from build123d import *

# Parameters (mm, degrees)
SKETCH1_R           = 34
BOSS_EXTRUDE1_DEPTH = 26.5
SKETCH2_R           = 23.2
CUT_EXTRUDE1_DEPTH  = 6.5
CUT_EXTRUDE1_DRAFT  = -66
SKETCH3_R           = 5.75
BOSS_EXTRUDE2_DEPTH = 5


with BuildPart() as part:
    # Sketch1 → Boss-Extrude1 (new body)
    with BuildSketch(Plane.XY):
        Circle(SKETCH1_R)
    extrude(amount=BOSS_EXTRUDE1_DEPTH)


with BuildPart() as cut_extrude1_tool:
    # Sketch2 → Cut-Extrude1 (with draft: the straight prism first)
    with BuildSketch(Plane.XY.offset(26.5)):
        Circle(SKETCH2_R)
    extrude(amount=-CUT_EXTRUDE1_DEPTH)
    # Cut-Extrude1: the draft: its side faces are tilted about the plane it starts from
    cut_extrude1_sides = [cut_extrude1_tool.faces().sort_by_distance(p)[0] for p in [
        (-23.2, 0, 23.25),
    ]]
    draft(cut_extrude1_sides, Plane.XY.offset(26.5), CUT_EXTRUDE1_DRAFT)


with BuildPart() as part_1:
    add(part.part)

    # Cut-Extrude1: cut by cut_extrude1_tool
    add(cut_extrude1_tool.part, mode=Mode.SUBTRACT)

    # Sketch3 → Boss-Extrude2 (add)
    with BuildSketch(Plane(origin=(0, 0, 0), x_dir=(-1, 0, 0), z_dir=(0, 0, -1))):
        Circle(SKETCH3_R)
    extrude(amount=BOSS_EXTRUDE2_DEPTH)


solid = part_1.part
Geometry check sheet. Reference: the model listing, model coordinates, mm. Coordinates: 2 decimals unless noted, no trailing zeros. Loops run counter-clockwise (first coordinate to the right, second up) from the corner with the lowest first, then second, coordinate; pieces in that order, holes last. Notation, with made-up numbers: (16.5, 42) - (23.5, 42) arc R23 ccw to (23.5, 71) - close; hole circle Ø4 at (-17, 1.25). An arc over 180 degrees is marked (long way). Use one line per item in the form item = value. Start each with the question number.
Item 1: Section check A-A, the plane y = 0. Enter the section's corners in (x, z).
Item 2: Thickness scan on probe 1 along Z at (x, y) = (-4, -25); probe 2 along Y at (x, z) = (1, 24.5); probe 3 along Y at (x, z) = (-0.5, 3.5). Record the ranges inside material, lowest first.
Item 3: Gauge pin test, flat ends, axial feed: pin 1 (8 mm diameter, centred on x = 6.5, z = 14.5, fed in from +Y); pin 2 (1 mm diameter, centred on y = 3, z = 9, fed in from -X); pin 3 (8 mm diameter, centred on y = 12, z = -1.5, fed in from -X). Record the tip position at first contact, or that the pin passes through.
Item 4: Mould release check, pull along X, two halves, no side actions. Record for faces 1 (the face through (0.75, 5.7, -2.46)), 2 (the face through (0, 0, -5)), 3 (the face through (0, 0, 20)): +X half, -X half, draft (parallel to the pull), parting line (faces both ways), or undercut.
Item 5: Section check C-C, the plane z = 19. Enter the section's corners in (x, y).
Item 6: Section check D-D, the plane y = -26.5. Enter the section's corners in (x, z), and give its area (3 significant figures).
Computed:
q1.outline = (-34, 0) - (-5.75, 0) - (-5.75, -5) - (5.75, -5) - (5.75, 0) - (34, 0) - (34, 26.5) - (23.2, 26.5) - (8.6, 20) - (-8.6, 20) - (-23.2, 26.5) - (-34, 26.5) - close
q2.probe_1 = 0 to 26.5
q2.probe_2 = -33.99 to -18.68, 18.68 to 33.99
q2.probe_3 = -34 to 34
q3.pin_1 = 33.91
q3.pin_2 = -33.91
q3.pin_3 = -32.97
q4.face_1 = parting line
q4.face_2 = draft
q4.face_3 = undercut
q5.outline = circle Ø68 at (0, 0)
q6.outline = (-21.3, 0) - (21.3, 0) - (21.3, 26.5) - (-21.3, 26.5) - close
q6.area = 1,130 mm2
